Could you check a few things on this model? Use its own coordinates, in mm. A direction names the side the tool comes from. Round coordinates to 2 decimals unless told otherwise and drop trailing zeros. Loops run counter-clockwise (first coordinate to the right, second up) from the corner with the lowest first, then second, coordinate; pieces in that order, holes last. Notation, with made-up numbers: (62.5, 63.5) - (101.5, 63.5) arc R24 ccw to (101.5, 85.5) - close; hole circle Ø3 at (26.25, 5.25). An arc over 180 degrees is marked (long way). Answer as CSV lines item,"result". Start each with the question number.
1) Suppose I cut it at A-A, the plane x = 58. Write out the boundary of the cut face in (y, z), then the cut area to 3 significant figures.
2) Suppose I cut it at B-B, the plane z = -38. Write out the boundary of the cut face in (x, y).
3) Suppose I cut it at C-C, the plane x = -2.5. Write out the boundary of the cut face in (y, z).
4) I'm going to push flat-ended pins straight in: pin 1 Ø4.5 at (x, z) = (28, -12.5) entering from -Y; pin 2 Ø8 at (x, y) = (74, -5.5) entering from -Z; pin 3 Ø2.5 at (x, z) = (67.5, -9) entering from +Y. Where does each tip first touch, or does it pass through?
5) Please list where these lines run through material, in increasing order: line 1 along Z through (x, y) = (29.5, 0); line 2 along X through (y, z) = (1.75, -31.5); line 3 along Y through (x, z) = (64, -10).
6) Which directions (+Z, -Z, +X, -X, +Y, -Y) give clear straight access to the entire face, cutting with the end or side of a thin tool? Please do faces 4 (the face through (49, -4.5, -10)), 5 (the face through (100, 0, -9)), 6 (the face through (103, 0, -15)).
7) We'd pull the mould along Y, two halves only. Please class faces 1 (the face through (53.24, -0.59, 4.46)), 2 (the face through (-20, 7.5, -31)), 3 (the face through (0, 0, -38)): pulls with the +Y half, pulls with the -Y half, needs draft (parallel to the pull), parting line crosses it, or undercut.
```python
from build123d import *

# Parameters (mm, degrees)
F1_DEPTH = 103
F2_DEPTH = 100
F0_R     = 4.5
F3_DEPTH = 108
F4_R     = 2
F7_DEPTH = 40


# Not quite as in the source:
# - a fillet or chamfer that OpenCascade refuses, or shapes differently, is made with other operations: its cross-section is extruded or revolved along the edge and cut away or added
# - after a boolean that leaves OpenCascade's solid faulty, fix() repairs it


with BuildPart() as f1:
    # F0 (on Right) → F1 (new body)
    with BuildSketch(Plane.YZ):
        with BuildLine():
            ThreePointArc((4.5, -15), (0, -10.5), (-4.5, -15))
            ThreePointArc((-4.5, -15), (0, -19.5), (4.5, -15))
        make_face()
    extrude(amount=F1_DEPTH)

    # F0 (on Right) → F2 (join)
    with BuildSketch(Plane.YZ):
        with BuildLine():
            ThreePointArc((4.5, -6), (0, -7.5), (-4.5, -6))
            Line((-4.5, -6), (-4.5, -15))
            ThreePointArc((-4.5, -15), (0, -10.5), (4.5, -15))
            Line((4.5, -15), (4.5, -6))
        make_face()
    extrude(amount=F2_DEPTH)

    # F0 (on Right) → F3 (join)
    with BuildSketch(Plane.YZ):
        with BuildLine():
            ThreePointArc((4.5, -6), (6.7082039325, -3.3541019662), (7.5, 0))
            ThreePointArc((7.5, 0), (-3.3541019662, 6.7082039325), (-4.5, -6))
            ThreePointArc((-4.5, -6), (0, -7.5), (4.5, -6))
        make_face()
        Circle(F0_R, mode=Mode.SUBTRACT)
    extrude(amount=F3_DEPTH)

    # F4
    f4_edges = [f1.edges().sort_by_distance(p)[0] for p in [
        (108, 4.5, 6),
    ]]
    fillet(f4_edges, radius=F4_R)

    # F5: fillet of radius 2 on 1 edges, made by hand

    # F5_s1 → F5_t2 (revolve, cut)
    with BuildSketch(Plane.XY.offset(-15)):
        with BuildLine():
            ThreePointArc((101, 4.5), (102.4142135624, 3.9142135624), (103, 2.5))
            Line((103, 2.5), (103, 4.5))
            Line((103, 4.5), (101, 4.5))
        make_face()
    revolve(axis=Axis((103, 0, -15), (-1, 0, 0)), mode=Mode.SUBTRACT)

    # F6 (on Right) → F7 (join)
    with BuildSketch(Plane.YZ):
        with BuildLine():
            ThreePointArc((-7.5, -60.5), (-6.9142135624, -61.9142135624), (-5.5, -62.5))
            Line((-5.5, -62.5), (5.5, -62.5))
            ThreePointArc((5.5, -62.5), (6.9142135624, -61.9142135624), (7.5, -60.5))
            Line((7.5, -60.5), (7.5, 0))
            ThreePointArc((7.5, 0), (5.3033008589, 5.3033008589), (0, 7.5))
            ThreePointArc((0, 7.5), (-5.3033008589, 5.3033008589), (-7.5, 0))
            Line((-7.5, 0), (-7.5, -60.5))
        make_face()
    extrude(amount=-F7_DEPTH)

    add(f1.part.fix(), mode=Mode.REPLACE)


solid = f1.part
```
Filled sheet:
1,outline,"(-4.5, -15) arc R4.5 ccw to (4.5, -15) - (4.5, -6) arc R7.5 ccw (long way) to (-4.5, -6) - close; hole circle Ø9 at (0, 0)"
1,area,"217 mm²"
2,outline,"(-40, -7.5) - (0, -7.5) - (0, 7.5) - (-40, 7.5) - close"
3,outline,"(-7.5, -60.5) arc R2 ccw to (-5.5, -62.5) - (5.5, -62.5) arc R2 ccw to (7.5, -60.5) - (7.5, 0) arc R7.5 ccw to (-7.5, 0) - close"
4,pin 1,"y = -4.5"
4,pin 2,"z = -19.24"
4,pin 3,"y = 4.5"
5,line 1,"-19.5 to -4.5, 4.5 to 7.5"
5,line 2,"-40 to 0"
5,line 3,"-4.5 to 4.5"
6,face 4,"-Z, +X, -Y"
6,face 5,"+X"
6,face 6,"-Z, +X, +Y, -Y"
7,face 1,"undercut"
7,face 2,"pulls with the +Y half"
7,face 3,"needs draft"
